Build history of the part. All positions in model axes, mm. Face numbers are marked on the shaded views. A direction names the side the tool comes from. Give positions to 0.01 mm unless a question says otherwise; leave off trailing zeros. Write each loop counter-clockwise with the first axis right and the second up, starting at its lowest first coordinate (ties: lowest second). Pieces come first, ordered by that corner, then holes.
from build123d import *

# Parameters (mm, degrees)
SKETCH1_W      = 6.8
SKETCH1_H      = 8
EXTRUDE1_DEPTH = 10
EXTRUDE2_DEPTH = 7.8
EXTRUDE3_DEPTH = 11
SKETCH4_R      = 15.011245784
EXTRUDE4_DEPTH = 11


with BuildPart() as part:
    # Sketch1 → Extrude1 (new body)
    with BuildSketch(Plane(origin=(0, 0, 0), x_dir=(1, 0, 0), z_dir=(0, 1, 0))):
        Rectangle(SKETCH1_W, SKETCH1_H)
    extrude(amount=EXTRUDE1_DEPTH)

    # Sketch2 → Extrude2 (cut, through all)
    with BuildSketch(Plane(origin=(3.4, 0, 0), x_dir=(0, 0, -1), z_dir=(1, 0, 0))):
        Polygon((4, 10), (-4, 0), (-4, 10), align=None)
    extrude(amount=-EXTRUDE2_DEPTH, mode=Mode.SUBTRACT)

    # Sketch3 → Extrude3 (cut, through all)
    with BuildSketch(Plane.XZ):
        with BuildLine():
            Line((1.15, 1.5), (1.15, -1.5))
            ThreePointArc((1.15, -1.5), (0, -2.65), (-1.15, -1.5))
            Line((-1.15, -1.5), (-1.15, 1.5))
            ThreePointArc((-1.15, 1.5), (0, 2.65), (1.15, 1.5))
        make_face()
    extrude(amount=-EXTRUDE3_DEPTH, mode=Mode.SUBTRACT)

    # Sketch4 → Extrude4 (cut, through all)
    with BuildSketch(Plane.XZ):
        with Locations((0, -18.621131967)):
            Circle(SKETCH4_R)
    extrude(amount=-EXTRUDE4_DEPTH, mode=Mode.SUBTRACT)


solid = part.part
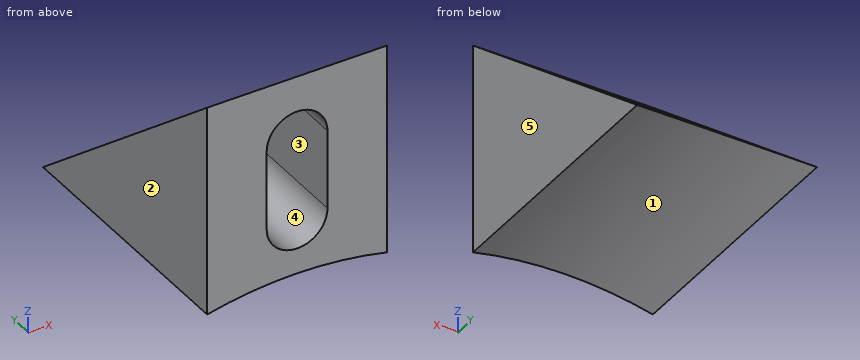
1. Saw through at B-B on x = 1. Give the cut face in (y, z).
2. 3-axis set-ups, long thin cutter, end or side, ignore diameter. For the marked faces 4 and 5: which of +Z, -Z, +X, -X, +Y, -Y reach the whole face in a straight line?
3. Saw through at A-A on z = -1. Give the cut face in (x, y), plus the area to 3 significant figures.
4. Drill centre lines: line 1 along X through (y, z) = (1.5, 1.5); line 2 along Z through (x, y) = (0, 2.25). Where is each one in solid material? Low to high.
5. Saw through at C-C on y = 5. Give the cut face in (x, z).
6. Saw through at D-D on z = 2.5. Give the cut face in (x, y) (3 decimals).
7. Drop a flat-ended pin along its axis: pin 1 (1 mm diameter, centred on y = 4, z = 3, fed in from -X). Give the stop position or say it passes through.
8. Mould opens along Z. For the marked faces 1, 2 and 3 say: pulls with the +Z half, pulls with the -Z half, needs draft (parallel to the pull), parting line crosses it, or undercut.
Outcome:
1. outline: (0, -3.64) - (9.55, -3.64) - (7.58, -2.07) - (0, -2.07) - close; (0, 2.07) - (2.42, 2.07) - (0, 4) - close
2. face 4: +Y, -Y
2. face 5: +Z, -Z, +X, +Y, -Y
3. outline: (-3.4, 0) - (-1.15, 0) - (-1.15, 6.25) - (-3.4, 6.25) - close; (1.15, 0) - (3.4, 0) - (3.4, 6.25) - (1.15, 6.25) - close
3. area: 28.1 mm2
4. line 1: x = -3.4 to -1.15, 1.15 to 3.4
4. line 2: z = -3.61 to -2.65
5. outline: (-3.4, -4) arc R15.01 cw to (3.4, -4) - (3.4, 0) - (1.15, 0) - (1.15, -1.5) arc R1.15 cw to (-1.15, -1.5) - (-1.15, 0) - (-3.4, 0) - close
6. outline: (-3.4, 0) - (-0.568, 0) - (-0.568, 1.875) - (-3.4, 1.875) - close; (0.568, 0) - (3.4, 0) - (3.4, 1.875) - (0.568, 1.875) - close
7. pin 1: passes through
8. face 1: pulls with the -Z half
8. face 2: needs draft
8. face 3: undercut
